from build123d import *

# Parameters (mm, degrees)
F1_DEPTH = 29
F2_R     = 2.75
F3_DEPTH = 50
F4_R     = 2.75
F5_DEPTH = 50


with BuildPart() as f1:
    # F0 (on Front) → F1 (new body)
    with BuildSketch(Plane.XZ):
        with BuildLine():
            ThreePointArc((-13.75, 0), (0, 13.75), (13.75, 0))
            Line((13.75, 0), (36.25, 0))
            Line((36.25, 0), (36.25, 30))
            Line((36.25, 30), (-36.25, 30))
            Line((-36.25, 30), (-36.25, 0))
            Line((-36.25, 0), (-13.75, 0))
        make_face()
    extrude(amount=F1_DEPTH)

    # F2 (on face) → F3 (cut)
    with BuildSketch(Plane.XY.offset(30)):
        with Locations((-18.75, -14.5)):
            Circle(F2_R)
        with Locations((18.75, -14.5)):
            Circle(F2_R)
    extrude(amount=-F3_DEPTH, mode=Mode.SUBTRACT)

    # F4 (on face) → F5 (cut)
    with BuildSketch(Plane.XZ.offset(29)):
        with Locations((-28.75, 15)):
            Circle(F4_R)
        with Locations((0, 22.5)):
            Circle(F4_R)
        with Locations((28.75, 15)):
            Circle(F4_R)
    extrude(amount=-F5_DEPTH, mode=Mode.SUBTRACT)


solid = f1.part
For this review, take the finished solid that the model builds, in its own axes (mm). Round coordinates to 2 decimals unless told otherwise and drop trailing zeros. Loops run counter-clockwise (first coordinate to the right, second up) from the corner with the lowest first, then second, coordinate; pieces in that order, holes last. Notation, with made-up numbers: (70, -37) - (92, -37) arc R35 ccw to (92, 1) - close; hole circle Ø3 at (-10, -24.5). An arc over 180 degrees is marked (long way). Put each result on its own line as item: value. Start each with the question number.
1. Mouldability with a two-part tool opening along Z and no side actions: class faces 1 (the flat face through (-25, -14, 0)), 2 (the flat face through (-1, -29, 15)), 3 (the cylindrical face through (26, -15, 15)), 4 (the cylindrical face through (-31.5, -14.7, 15.1)) as +Z half, -Z half, draft (parallel to the pull), parting line (faces both ways), or undercut.
2. Consider section A-A on x = 18.75. State the section outline as (y, z) points, plus the area to 3 significant figures.
3. Consider section B-B on y = -15.5. State the section outline as (x, z) points.
4. For probe 1 along Y at (x, z) = (18.75, 23.5); probe 2 along X at (y, z) = (-21.25, 6.25); probe 3 along Z at (x, y) = (-28.75, -18), list the stretches that pass through material, from the lowest coordinate up. Write a range as [from, to].
5. Consider section D-D on z = 3.5. State the section outline as (x, y) points.
6. Insertion check: P1, Ø12, axis at x = -4, y = -22.5, coming from the -Z side. The pin has a flat end and moves straight along its axis. Give the tip position at first contact, or say it passes through.
7. Consider section C-C on y = -7. State the section outline as (x, z) points.
Result sheet:
1. face 1: -Z half
1. face 2: draft
1. face 3: undercut
1. face 4: undercut
2. outline: (-29, 0) - (-17.25, 0) - (-17.25, 30) - (-29, 30) - close; (-11.75, 0) - (0, 0) - (0, 30) - (-11.75, 30) - close
2. area: 705 mm^2
3. outline: (-36.25, 0) - (-21.31, 0) - (-21.31, 30) - (-36.25, 30) - close; (-16.19, 0) - (-13.75, 0) arc R13.75 cw to (13.75, 0) - (16.19, 0) - (16.19, 30) - (-16.19, 30) - close; (21.31, 0) - (36.25, 0) - (36.25, 30) - (21.31, 30) - close; hole circle Ø5.5 at (-28.75, 15); hole circle Ø5.5 at (0, 22.5); hole circle Ø5.5 at (28.75, 15)
4. probe 1: [-29, -17.25], [-11.75, 0]
4. probe 2: [-36.25, -12.25], [12.25, 36.25]
4. probe 3: [0, 12.25], [17.75, 30]
5. outline: (-36.25, -29) - (-13.3, -29) - (-13.3, 0) - (-36.25, 0) - close; (13.3, -29) - (36.25, -29) - (36.25, 0) - (13.3, 0) - close; hole circle Ø5.5 at (-18.75, -14.5); hole circle Ø5.5 at (18.75, -14.5)
6. P1: z = 9.44
7. outline: (-36.25, 0) - (-13.75, 0) arc R13.75 cw to (13.75, 0) - (36.25, 0) - (36.25, 30) - (-36.25, 30) - close; hole circle Ø5.5 at (-28.75, 15); hole circle Ø5.5 at (0, 22.5); hole circle Ø5.5 at (28.75, 15)
